Work out the finished part from the listing and answer in its coordinate system (mm). A direction names the side the tool comes from. Round coordinates to 2 decimals unless told otherwise and drop trailing zeros. Write each loop counter-clockwise with the first axis right and the second up, starting at its lowest first coordinate (ties: lowest second). Pieces come first, ordered by that corner, then holes. Notation, with made-up numbers: (55.25, 75.5) - (98.25, 75.5) arc R30 ccw to (98.25, 97.5) - close; hole circle Ø9 at (-18, -30.75). An arc over 180 degrees is marked (long way). Write item = value, one per line. Start each with the question number.
from build123d import *

# Parameters (mm, degrees)
F1_DEPTH = 76.2
F2_R     = 2.54
F3_T     = 2.54


# Not quite as in the source:
# - a shell that OpenCascade refuses in one call is made with other operations: the cavity is built on its own and cut out


with BuildPart() as f1:
    # F0 (on Front) → F1 (new body)
    with BuildSketch(Plane.XZ):
        Polygon((16.1029547439, 16.1029547439), (0, 76.2), (0, 0), (76.2, 0), align=None)
    extrude(amount=F1_DEPTH)

    # F2
    f2_edges = [f1.edges().sort_by_distance(p)[0] for p in [
        (0, -38.1, 76.2),
        (76.2, -38.1, 0),
        (16.102955, -38.1, 16.102955),
        (0, -38.1, 0),
    ]]
    fillet(f2_edges, radius=F2_R)

    # F3: shell of thickness 2.54, made by hand


with BuildPart() as f3_core1:
    # F3_t2: copy of F1
    add(f1.part)

    # the walls: a layer under each face that stays
    f3_faces = [f3_core1.faces().sort_by_distance(p)[0] for p in [
        (10.3584280297, -38.1, 37.5418203066),
        (9.9077974256, 0, 9.9077974256),
        (16.3808048352, -38.1, 16.3808048352),
        (37.5418203066, -38.1, 10.3584280297),
        (0, -38.1, 29.7233922768),
        (29.7233922768, -38.1, 0),
    ]]
    thicken(f3_faces, amount=-F3_T, mode=Mode.SUBTRACT)


with BuildPart() as f1_1:
    add(f1.part)

    # what is left inside the walls is the cavity
    f3_cavity = [f3_core1.part.solids().sort_by_distance(p)[0] for p in [
        (29.723392, -51.646667, 2.5654),
    ]]
    add(f3_cavity, mode=Mode.SUBTRACT)


solid = f1_1.part
1. Find section A-A on y = -42.5. Give the vertices of the cut face in (x, z).
2. For a pull along Z with two mould halves and no side action, classify faces 1 (the face through (7.98, -38.85, 36.6)), 2 (the face through (10.434, -37.567, 37.262)), 3 (the face through (14.56, -39.89, 14.61)), 4 (the face through (0, -38, 30)) as released by +Z, released by -Z, zero draft, split by the parting line, or undercut.
3. Find section C-C on x = 37. Give the vertices of the cut face in (y, z), plus the area to 3 significant figures.
4. Find section B-B on z = 24.5. Give the vertices of the cut face in (x, y), plus the area to 3 significant figures.
5. Each of these flat-tipped pins is pushed along its axis until it touches: pin 1 (4 mm diameter, centred on x = 28.5, y = -42, fed in from +Z); pin 2 (8 mm diameter, centred on y = -51.5, z = 49.5, fed in from +X). Where does it stop, or does it pass through?
6. Consider line 1 (Y direction, x = 3.5, z = 51); line 2 (X direction, y = -33.5, z = 26); line 3 (Z direction, x = 29, y = -22). Determine where each line is inside the solid, lowest interval first.
7. Which of the six approach directions +Z, -Z, +X, -X, +Y, -Y give full straight-line access (tool end or side, diameter ignored) to faces 5 (the face through (2.26, -38.63, 59.43)), 6 (the face through (2.54, -39, 30))?
Answer key:
q1.outline = (0, 2.54) arc R2.54 ccw to (2.54, 0) - (56.91, 0) arc R2.54 ccw to (57.56, 4.99) - (17.52, 15.72) arc R2.54 cw to (15.72, 17.52) - (4.99, 57.56) arc R2.54 ccw to (0, 56.91) - close; hole (2.54, 2.54) - (56.91, 2.54) - (16.86, 13.27) arc R5.08 cw to (13.27, 16.86) - (2.54, 56.91) - close
q2.face_1 = undercut
q2.face_2 = released by +Z
q2.face_3 = undercut
q2.face_4 = zero draft
q3.outline = (-76.2, 0) - (0, 0) - (0, 10.5) - (-76.2, 10.5) - (-76.2, 7.87) - (-2.54, 7.87) - (-2.54, 2.54) - (-76.2, 2.54) - close
q3.area = 407 mm²
q4.outline = (0, -76.2) - (2.54, -76.2) - (2.54, -2.54) - (11.22, -2.54) - (11.22, -76.2) - (13.85, -76.2) - (13.85, 0) - (0, 0) - close
q4.area = 416 mm²
q5.pin_1 = 13.32
q5.pin_2 = 8.23
q6.line_1 = -2.54 to 0
q6.line_2 = 0 to 2.54, 10.82 to 13.45
q6.line_3 = 0 to 2.54, 10.02 to 12.65
q7.face_5 = +Z, +Y, -Y
q7.face_6 = -Y
